Model file for the job. Use its own axes, mm. A direction names the side the tool comes from. Round coordinates to 2 decimals unless told otherwise and drop trailing zeros. Loops run counter-clockwise (first coordinate to the right, second up) from the corner with the lowest first, then second, coordinate; pieces in that order, holes last. Notation, with made-up numbers: M 79.5,-37 L 83.5,-37 A18 ccw 83.5,-25 Z; hole C 9.5,38.25 d8. An arc over 180 degrees is marked long. Use a Markdown table: item, result. Add a question column.
Q1. Probe line 1 (X direction, y = 305, z = -72); line 2 (X direction, y = 429, z = -33.5); line 3 (Y direction, x = 194, z = -144.5). List the from-to ranges inside material, lowest first. Write a range as from..to.
Q2. Tool access for faces 1 (the face through (-8, 0, 0)), 2 (the face through (-1, 504, -378.628)): list every direction of +Z, -Z, +X, -X, +Y, -Y with a clear straight run to the whole face (end or side of a thin tool).
Q3. Pin check, flat tips, straight feed: pin 1 (16 mm diameter, centred on y = 139.5, z = -1.5, fed in from +X); pin 2 (1.5 mm diameter, centred on y = 358.5, z = -119.5, fed in from +X); pin 3 (0.5 mm diameter, centred on y = 514, z = -378.5, fed in from +X); pin 4 (10 mm diameter, centred on x = 337.5, z = -184, fed in from -Y). Stop position of each tip, or through.
Q4. Cut at B-B (y = 507.5). Give the cut face in (x, z).
Q5. Cut at A-A (x = 24.5). Give the cut face in (y, z) (1 decimal), plus the area to 3 significant figures.
from build123d import *

# Parameters (mm, degrees)
SKETCH1_W               = 1088
SKETCH1_H               = 20
BOSS_EXTRUDE1_DEPTH     = 1
BOSS_EXTRUDE4_DEPTH     = 1088
SKETCH5_W               = 1088
SKETCH5_H               = 1
BOSS_EXTRUDE5_DEPTH     = 582
BOSS_EXTRUDE6_DEPTH     = 1088
SKETCH7_W               = 148
SKETCH7_H               = 1
BOSS_EXTRUDE7_DEPTH     = 106
CUT_EXTRUDE3_DEPTH      = 148
SKETCH13_W              = 470
SKETCH13_H              = 1
CUT_REVOLVE1_ANGLE      = 39.3
BOSS_EXTRUDE11_DEPTH    = 748.0802096
BOSS_EXTRUDE12_DEPTH    = 800
SKETCH18_W              = 570.021392147
SKETCH18_H              = 387.152750426
CUT_EXTRUDE5_DEPTH      = 1477.790454702
CUT_EXTRUDE6_DEPTH      = 800
CUT_EXTRUDE6_DEPTH_BACK = 10
BOSS_EXTRUDE13_DEPTH    = 748.0802096
BOSS_EXTRUDE14_DEPTH    = 748.0802096
SKETCH21_W              = 476.858853826
SKETCH21_H              = 325.647229621
CUT_EXTRUDE7_DEPTH      = 1432.718358443
CUT_EXTRUDE9_DEPTH      = 10
CUT_EXTRUDE9_DEPTH_BACK = 946.037072047
BOSS_EXTRUDE15_DEPTH    = 20
FILLET1_R               = 10
BOSS_EXTRUDE20_DEPTH    = 20
FILLET2_R               = 10


with BuildPart() as part:
    # Sketch1 → Boss-Extrude1 (new body)
    with BuildSketch(Plane(origin=(0, 0, 0), x_dir=(1, 0, 0), z_dir=(0, 1, 0))):
        Rectangle(SKETCH1_W, SKETCH1_H)
    extrude(amount=BOSS_EXTRUDE1_DEPTH)

    # Sketch4 → Boss-Extrude4 (add)
    with BuildSketch(Plane.ZY.offset(544)):
        with BuildLine():
            Line((-10, 1), (-10.77384021, 0.366619127))
            ThreePointArc((-10.77384021, 0.366619127), (-10.428146661, 0.096290735), (-10, 0))
            Line((-10, 0), (-10, 1))
        make_face()
    extrude(amount=-BOSS_EXTRUDE4_DEPTH)

    # Sketch5 → Boss-Extrude5 (add)
    with BuildSketch(Plane(origin=(0, 5.500184543, -4.501848885), x_dir=(1, 0, 0), z_dir=(0, 0.7738402097265025, -0.6333808726275548))):
        with Locations((0, 7.605021225)):
            Rectangle(SKETCH5_W, SKETCH5_H)
    extrude(amount=BOSS_EXTRUDE5_DEPTH)

    # Sketch6 → Boss-Extrude6 (add)
    with BuildSketch(Plane(origin=(544, 0, 0), x_dir=(0, 0, -1), z_dir=(1, 0, 0))):
        with BuildLine():
            Line((378.627667869, 451.375002061), (379.627667869, 451.375002061))
            ThreePointArc((379.627667869, 451.375002061), (379.569432227, 451.038728519), (379.401508079, 450.741621188))
            Line((379.401508079, 450.741621188), (378.627667869, 451.375002061))
        make_face()
    extrude(amount=-BOSS_EXTRUDE6_DEPTH)

    # Sketch7 → Boss-Extrude7 (add)
    with BuildSketch(Plane(origin=(0, 451.375002061, 0), x_dir=(1, 0, 0), z_dir=(0, 1, 0))):
        with Locations((0, 379.127667869)):
            Rectangle(SKETCH7_W, SKETCH7_H)
    extrude(amount=BOSS_EXTRUDE7_DEPTH)

    # Sketch8 → Cut-Extrude3 (cut)
    with BuildSketch(Plane(origin=(0, -4.500184543, -5.498151115), x_dir=(1, 0, 0), z_dir=(0, 0.6333808726275547, 0.7738402097265025))):
        Polygon((74, 589.107648936), (544, 7.107648936), (544, 589.107648936), align=None)
        Polygon((-74, 589.107648936), (-544, 7.107648936), (-544, 589.107648936), align=None)
    extrude(amount=-CUT_EXTRUDE3_DEPTH, mode=Mode.SUBTRACT)

    # Sketch13 → Cut-Revolve1 (revolve, cut)
    with BuildSketch(Plane(origin=(0, 451.375002061, 0), x_dir=(1, 0, 0), z_dir=(0, 1, 0))):
        with Locations((309, 379.127667869)):
            Rectangle(SKETCH13_W, SKETCH13_H)
        with Locations((-309, 379.127667869)):
            Rectangle(SKETCH13_W, SKETCH13_H)
    revolve(axis=Axis((-544, 451.375002061, -378.627667869), (-1, 0, 0)), revolution_arc=CUT_REVOLVE1_ANGLE, mode=Mode.SUBTRACT)

    # 3DSketch8 → Boss-Extrude11 (add)
    with BuildSketch(Plane(origin=(-74, 450.741621188, -379.401508079), x_dir=(0, 0.6333808726023494, 0.7738402097471327), z_dir=(-0.6282748747614416, -0.602041059623436, 0.49276489756372194))):
        with BuildLine():
            Line((0, 0), (1, 0))
            Line((1, 0), (0.393252863, 0.794894906))
            ThreePointArc((0.393252863, 0.794894906), (0.103688911, 0.443425791), (0, 0))
        make_face()
    extrude(amount=BOSS_EXTRUDE11_DEPTH)

    # Sketch17 → Boss-Extrude12 (add)
    with BuildSketch(Plane(origin=(-119.830134924, 202.692581564, 94.858610661), x_dir=(0.8810391406721232, 0.4420570737301439, 0.16839114041085765), z_dir=(-0.4720440788324485, 0.7984621982715473, 0.37367433089602736))):
        Polygon((69.885181219, 532.84001368), (70.561407095, 532.10331933), (70.579071373, 532.119533725), (69.90284514, 532.856227747), align=None)
        Polygon((-481.203373087, 26.984765587), (-480.527146854, 26.248071566), (70.561407095, 532.10331933), (69.885181219, 532.84001368), align=None)
    extrude(amount=BOSS_EXTRUDE12_DEPTH)

    # Sketch18 → Cut-Extrude5 (cut, through all)
    with BuildSketch(Plane(origin=(0, 1, 0), x_dir=(1, 0, 0), z_dir=(0, 1, 0))):
        with Locations((-773.718733555, -183.576375213)):
            Rectangle(SKETCH18_W, SKETCH18_H)
    extrude(amount=CUT_EXTRUDE5_DEPTH, mode=Mode.SUBTRACT)

    # 3DSketch9 → Cut-Extrude6 (cut, two sides: drawn at the far end of the back side and taken through both)
    with BuildSketch(Plane(origin=(-74, 450.741621188, -379.401508079), x_dir=(-0.7561274717373775, 0.6544243626913974, 3.634948491477008e-14), z_dir=(0, 0, 1)).offset(-CUT_EXTRUDE6_DEPTH_BACK)):
        Polygon((0, 0), (591.099614486, 511.59361742), (1033.881208267, 0), (442.781593781, -511.59361742), align=None)
    extrude(amount=CUT_EXTRUDE6_DEPTH + CUT_EXTRUDE6_DEPTH_BACK, mode=Mode.SUBTRACT)

    # 3DSketch11 → Boss-Extrude13 (add)
    with BuildSketch(Plane(origin=(74, 450.741621188, -379.401508079), x_dir=(0, 0.6333808726276229, 0.7738402097264466), z_dir=(-0.6282748747614613, 0.60204105960733, -0.4927648975833744))):
        with BuildLine():
            Line((0, 0), (1, 0))
            Line((1, 0), (0.391238571, 0.79335334))
            ThreePointArc((0.391238571, 0.79335334), (0.103127258, 0.44228869), (0, 0))
        make_face()
    extrude(amount=-BOSS_EXTRUDE13_DEPTH)

    # Sketch20 → Boss-Extrude14 (add)
    with BuildSketch(Plane(origin=(120.641152421, 203.389944625, 94.67657513), x_dir=(0.8807290157776859, -0.4307943838243474, -0.19680599491039222), z_dir=(0.47361118117402395, 0.7984651172491827, 0.37167984287985667))):
        Polygon((-54.061283152, 534.279462102), (-54.759673843, 533.563745369), (480.649426942, 11.115806908), (481.347817633, 11.831523641), align=None)
    extrude(amount=BOSS_EXTRUDE14_DEPTH)

    # Sketch21 → Cut-Extrude7 (cut, through all)
    with BuildSketch(Plane(origin=(0, 1, 0), x_dir=(1, 0, 0), z_dir=(0, 1, 0))):
        with Locations((750.93268392, -152.823614809)):
            Rectangle(SKETCH21_W, SKETCH21_H)
    extrude(amount=CUT_EXTRUDE7_DEPTH, mode=Mode.SUBTRACT)

    # 3DSketch12 → Cut-Extrude9 (cut, two sides: drawn at the far end of the back side and taken through both)
    with BuildSketch(Plane(origin=(74, 450.741621188, -379.401508079), x_dir=(0.7338585271859536, 0.6793023348086353, 3.7729204364225037e-14), z_dir=(0, 0, -1)).offset(-CUT_EXTRUDE9_DEPTH_BACK)):
        Polygon((0, 0), (611.708587654, 566.233213109), (1135.847136792, 0), (524.138549137, -566.233213109), align=None)
    extrude(amount=CUT_EXTRUDE9_DEPTH + CUT_EXTRUDE9_DEPTH_BACK, mode=Mode.SUBTRACT)

    # Sketch23 → Boss-Extrude15 (add)
    with BuildSketch(Plane.XY.offset(-10.000000002)):
        Polygon((543.999997701, 1.01026286), (543.899342545, 450.741621188), (544.899342545, 450.741845), (544.999997701, 1.010486671), align=None)
    extrude(amount=BOSS_EXTRUDE15_DEPTH)

    # Fillet1
    # the kernel refuses this fillet: 10 mm, written as the material it takes off along each edge
    with BuildSketch(Plane(origin=(545.517698589, 458.812119138, -10.000000002), x_dir=(-0.7867889291912172, -0.0001760925956154425, -0.6172221236261185), z_dir=(0.00022381172976857925, -0.9999999749541545, 0))) as fillet1_piece_1:
        with BuildLine():
            CenterArc((3.228199261, -10), FILLET1_R, 90, 15.90399317)
            Line((0.487936805, -0.382777861), (0, 0))
            Line((0, 0), (3.228199261, 0))
        make_face()
    extrude(amount=464.182000108, mode=Mode.SUBTRACT)

    # Sketch26 → Boss-Extrude20 (add)
    with BuildSketch(Plane.XY.offset(-10)):
        Polygon((-542.426656099, 450.741621188), (-543.999929799, 1.020067072), (-544.999929799, 1.023565401), (-543.426656099, 450.745119517), align=None)
    extrude(amount=BOSS_EXTRUDE20_DEPTH)

    # Fillet2
    # the kernel refuses this fillet: 10 mm, written as the material it takes off along each edge
    with BuildSketch(Plane(origin=(-544.015507205, 458.793802403, -10), x_dir=(0.7858388463706936, -0.0027491223803662495, -0.618425217678674), z_dir=(-0.003498307026844443, -0.9999938809052514, 0))) as fillet2_piece_1:
        with BuildLine():
            CenterArc((3.220892195, 10), FILLET2_R, 254.121260496, 15.878739504)
            Line((0.484868888, 0.381570998), (0, 0))
            Line((0, 0), (3.220892195, 0))
        make_face()
    extrude(amount=464.167480485, mode=Mode.SUBTRACT)


solid = part.part
Checked values:
| question | item | result |
|---|---|---|
| 1 | line 1 | x = -465.77..-464.15, 464.9..466.52 |
| 1 | line 2 | x = -514.26..-512.64, 513.95..515.57 |
| 1 | line 3 | y = 163.75..165.33 |
| 2 | face 1 | +Z, -Z, +X, -X, -Y |
| 2 | face 2 | +Z, +X, -X, +Y |
| 3 | pin 1 | stops at x = 544.97 |
| 3 | pin 2 | stops at x = 406.91 |
| 3 | pin 3 | stops at x = 74 |
| 3 | pin 4 | passes through |
| 4 | outline | M -74,-379.63 L 74,-379.63 L 74,-378.63 L -74,-378.63 Z |
| 5 | outline | M 0,-10 A1 ccw 0.4,-10.8 L 450.7,-379.4 A1 ccw 451.4,-379.6 L 557.4,-379.6 L 557.4,-378.6 L 451.4,-378.6 L 1,-10 L 1,10 L 0,10 Z |
| 5 | area | 709 mm^2 |
